Source: CAD feature listing. Evaluate the final solid. Frame: model axes, mm. A direction names the side the tool comes from. Round coordinates to 2 decimals unless told otherwise and drop trailing zeros. Loops run counter-clockwise (first coordinate to the right, second up) from the corner with the lowest first, then second, coordinate; pieces in that order, holes last.
Item 1: Access query for faces 1 (the flat face through (3, 2, 0)), 2 (the flat face through (0, 9, 13.5)), 3 (the flat face through (9, 5, 0)). Directions: +Z, -Z, +X, -X, +Y, -Y. A direction counts if a zero-diameter tool reaches every point of the face in a straight line with its end or side. Return the directions, or none.
Item 2: First-contact query: P1, Ø1.8, axis at x = -1, z = 0, coming from the -Y side; P2, Ø5, axis at x = 0, z = 0.5, coming from the +Y side. Flat tips, straight axial feed; report the tip coordinate or a pass-through.
Item 3: Section query D-D on y = 7.5. Return loops of the section in (x, z).
Item 4: Section query B-B on x = -0.75. Return loops of the section in (y, z), then the cut area to 3 significant figures.
Item 5: Section query C-C on z = -4.25. Return loops of the section in (x, y).
Item 6: Section query A-A on y = 1.25. Return loops of the section in (x, z).
Item 7: Ray query, L1, parallel to Z at x = 1.25, y = 2.25; L2, parallel to Z at x = 6, y = 8.5; L3, parallel to X at y = 3.25, z = 1. Return the intervals inside material, ascending.
Autodesk Inventor part; units mm, degrees
ref_plane "YZ Plane" through (0, 0, 0) normal (1, 0, 0) x (0, 1, 0)
ref_plane "XZ Plane" through (0, 0, 0) normal (0, 1, 0) x (-1, 0, 0)
ref_plane "XY Plane" through (0, 0, 0) normal (0, 0, 1) x (1, 0, 0)
sketch "Sketch1" plane through (0, 0, 0) normal (0, 1, 0) x (-1, 0, 0)
  line L0 (9, 15) -> (-9, 15)
  line L1 (-9, 15) -> (-9, -15)
  line L2 (-9, -15) -> (9, -15)
  line L3 (9, -15) -> (9, 15)
  point P0 (0, 0)
  dimension "d0" = 30
  dimension "d1" = 18
  dimension "d7" = 15
  dimension "d8" = 9
extrude "Extrusion1" add sketch "Sketch1" along normal blind 11
sketch "Sketch2" plane through (0, 11, 0) normal (0, 1, 0) x (1, 0, 0)
  line L0 (-8.25, -13.5) -> (8.25, -13.5)
  line L1 (8.25, -13.5) -> (8.25, 13.5)
  line L2 (8.25, 13.5) -> (-8.25, 13.5)
  line L3 (-8.25, 13.5) -> (-8.25, -13.5)
  point P0 (0, 0)
  dimension "d4" = 27
  dimension "d5" = 16.5
  dimension "d6" = 13.5
  dimension "d9" = 8.25
extrude "Extrusion2" cut sketch "Sketch2" against normal blind 4
sketch "Sketch3" plane through (0, 0, 0) normal (0, -1, 0) x (1, 0, 0)
  line L0 (3, 3) -> (-3, 3)
  line L1 (-3, 3) -> (-3, -3)
  line L2 (-3, -3) -> (3, -3)
  line L3 (3, -3) -> (3, 3)
  point P0 (0, 0)
  dimension "d12" = 6
  dimension "d13" = 6
  dimension "d14" = 3
  dimension "d15" = 3
extrude "Extrusion3" cut sketch "Sketch3" against normal blind 5
properties part number "holder"
Data:
1. face 1: -Y
1. face 2: +Y
1. face 3: +Z, -Z, +X, +Y, -Y
2. P1: stops at y = 5
2. P2: stops at y = 7
3. outline: (-9, -15) - (9, -15) - (9, 15) - (-9, 15) - close; hole (-8.25, -13.5) - (8.25, -13.5) - (8.25, 13.5) - (-8.25, 13.5) - close
4. outline: (0, -15) - (11, -15) - (11, -13.5) - (7, -13.5) - (7, 13.5) - (11, 13.5) - (11, 15) - (0, 15) - (0, 3) - (5, 3) - (5, -3) - (0, -3) - close
4. area: 192 mm2
5. outline: (-9, 0) - (9, 0) - (9, 11) - (8.25, 11) - (8.25, 7) - (-8.25, 7) - (-8.25, 11) - (-9, 11) - close
6. outline: (-9, -15) - (9, -15) - (9, 15) - (-9, 15) - close; hole (-3, -3) - (3, -3) - (3, 3) - (-3, 3) - close
7. L1: z = -15 to -3, 3 to 15
7. L2: z = -15 to -13.5, 13.5 to 15
7. L3: x = -9 to -3, 3 to 9
